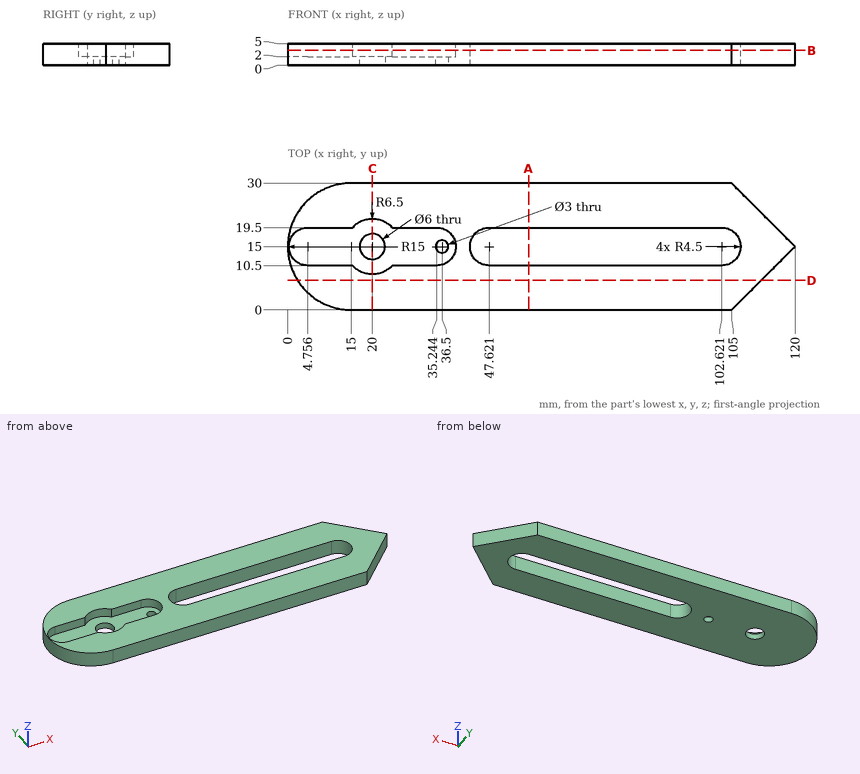
Input: dimensioned drawing with shaded views. Units: mm. Origin: part minimum x, y, z. Round coordinates to 2 decimals unless told otherwise and drop trailing zeros. Write each loop counter-clockwise with the first axis right and the second up, starting at its lowest first coordinate (ties: lowest second). Pieces come first, ordered by that corner, then holes. Notation, with made-up numbers: (35.25, 2) -> (76.25, 2) arc R23 ccw to (76.25, 39) -> close; hole circle Ø2 at (13, -31). An arc over 180 degrees is marked (long way). Use CSV: the item, a comma, the result in double quotes. Start each with the question number.
Q1. Section D-D (y = 7). Return loops of the section in (x, z).
Q2. Section A-A (x = 57). Return loops of the section in (y, z).
Q3. Section B-B (z = 3.5). Return loops of the section in (x, y) (1 decimal).
Q4. First-contact query: pin 1 Ø4 at (x, y) = (19.5, 18) entering from +Z; pin 2 Ø1.5 at (x, z) = (10, 4) entering from +Y (1 decimal). Flat tips, straight axial feed; report the tip coordinate or a pass-through.
Q5. Line query: L1, parallel to Y at x = 20, z = 1.4; L2, parallel to Y at x = 97, z = 1.25; L3, parallel to X at y = 12.5, z = 2.1 (1 decimal). Output: solid intervals per line, ascending.
Q6. Section C-C (x = 20). Return loops of the section in (y, z).
Result sheet:
1,outline,"(2.31, 0) -> (112, 0) -> (112, 5) -> (2.31, 5) -> close"
2,outline,"(0, 0) -> (10.5, 0) -> (10.5, 5) -> (0, 5) -> close; (19.5, 0) -> (30, 0) -> (30, 5) -> (19.5, 5) -> close"
3,outline,"(15, 0) -> (105, 0) -> (120, 15) -> (105, 30) -> (15, 30) arc R15 ccw to start; hole (4.8, 10.5) -> (15.3, 10.5) arc R6.5 ccw to (24.7, 10.5) -> (35.2, 10.5) arc R4.5 ccw to (35.2, 19.5) -> (24.7, 19.5) arc R6.5 ccw to (15.3, 19.5) -> (4.8, 19.5) arc R4.5 ccw to start; hole (47.6, 10.5) -> (102.6, 10.5) arc R4.5 ccw to (102.6, 19.5) -> (47.6, 19.5) arc R4.5 ccw to start"
4,pin 1,"z = 2"
4,pin 2,"y = 29.4"
5,L1,"0 to 12, 18 to 30"
5,L2,"0 to 10.5, 19.5 to 30"
5,L3,"0.2 to 1, 39 to 43.9, 106.4 to 117.5"
6,outline,"(0, 0) -> (12, 0) -> (12, 2) -> (8.5, 2) -> (8.5, 5) -> (0, 5) -> close; (18, 0) -> (30, 0) -> (30, 5) -> (21.5, 5) -> (21.5, 2) -> (18, 2) -> close"
